```python
from build123d import *

# Parameters (mm, degrees)
SKETCH_1_W          = 13.6
SKETCH_1_H          = 5
EXTRUDE_1_DEPTH     = 1.2
SKETCH_2_W          = 1.2
SKETCH_2_H          = 5
EXTRUDE_2_DEPTH     = 5
SKETCH_3_R          = 1
CUT_EXTRUDE_1_DEPTH = 14
SKETCH_5_W          = 1.2
SKETCH_5_H          = 5
EXTRUDE_3_DEPTH     = 2


with BuildPart() as part:
    # 草图1 → 凸台-拉伸1 (new body)
    with BuildSketch(Plane.XY):
        with Locations((8.287992891, 2.5)):
            Rectangle(SKETCH_1_W, SKETCH_1_H)
    extrude(amount=EXTRUDE_1_DEPTH)

    # 草图2 → 凸台-拉伸2 (add)
    with BuildSketch(Plane(origin=(0, 0, 1.2), x_dir=(-1, 0, 0), z_dir=(0, 0, -1))):
        with Locations((-14.487992891, 2.5)):
            Rectangle(SKETCH_2_W, SKETCH_2_H)
        with Locations((-2.087992891, 2.5)):
            Rectangle(SKETCH_2_W, SKETCH_2_H)
    extrude(amount=-EXTRUDE_2_DEPTH)

    # 草图3 → 切除-拉伸1 (cut)
    with BuildSketch(Plane(origin=(15.087992891, 0, 0), x_dir=(0, 0, -1), z_dir=(1, 0, 0))):
        with Locations((-4, 2.5)):
            Circle(SKETCH_3_R)
    extrude(amount=-CUT_EXTRUDE_1_DEPTH, mode=Mode.SUBTRACT)

    # 草图5 → 凸台-拉伸3 (add)
    with BuildSketch(Plane(origin=(0, 0, 0), x_dir=(-1, 0, 0), z_dir=(0, 0, -1))):
        with Locations((-2.087992891, 2.5)):
            Rectangle(SKETCH_5_W, SKETCH_5_H)
    extrude(amount=EXTRUDE_3_DEPTH)


solid = part.part
```
Build history of the part. All positions in model axes, mm. A direction names the side the tool comes from. Give positions to 0.01 mm unless a question says otherwise; leave off trailing zeros. Loops run counter-clockwise (first coordinate to the right, second up) from the corner with the lowest first, then second, coordinate; pieces in that order, holes last. Notation, with made-up numbers: (-14.5, 15.25) - (19.5, 15.25) arc R21 ccw to (19.5, 34.25) - close; hole circle Ø10 at (68.5, -12). An arc over 180 degrees is marked (long way). Use a Markdown table: item, result.
(1) Band-saw the part on A-A (y = 2.5). Give the cut face in (x, z), and give its area (3 significant figures).
Taken from the geometry:
| item | result |
|---|---|
| outline | (1.49, -2) - (2.69, -2) - (2.69, 0) - (15.09, 0) - (15.09, 3) - (13.89, 3) - (13.89, 1.2) - (2.69, 1.2) - (2.69, 3) - (1.49, 3) - close; (1.49, 5) - (2.69, 5) - (2.69, 6.2) - (1.49, 6.2) - close; (13.89, 5) - (15.09, 5) - (15.09, 6.2) - (13.89, 6.2) - close |
| area | 25.9 mm2 |
(2) Wall check: line 1 along X through (y, z) = (2.65, 2.5); line 2 along Y through (x, z) = (14.7, 4); line 3 along Z through (x, y) = (12.25, 0.3). Give the ranges that are in metal, low to high.
Taken from the geometry:
| item | result |
|---|---|
| line 1 | 1.49 to 2.69, 13.89 to 15.09 |
| line 2 | 0 to 1.5, 3.5 to 5 |
| line 3 | 0 to 1.2 |
(3) Band-saw the part on B-B (z = 4). Give the cut face in (x, y).
Taken from the geometry:
| item | result |
|---|---|
| outline | (1.49, 0) - (2.69, 0) - (2.69, 1.5) - (1.49, 1.5) - close; (1.49, 3.5) - (2.69, 3.5) - (2.69, 5) - (1.49, 5) - close; (13.89, 0) - (15.09, 0) - (15.09, 1.5) - (13.89, 1.5) - close; (13.89, 3.5) - (15.09, 3.5) - (15.09, 5) - (13.89, 5) - close |
(4) Which spindle directions (+Z, -Z, +X, -X, +Y, -Y) get a long thin tool onto all of the face, cutting with end or side? Do faces 1 (the face through (8, 3, 1.2)), 2 (the face through (15.088, 2, 2)), 3 (the face through (2.688, 2, -1)). Say none if no direction does.
Taken from the geometry:
| item | result |
|---|---|
| face 1 | +Z, +Y, -Y |
| face 2 | +Z, -Z, +X, +Y, -Y |
| face 3 | -Z, +X, +Y, -Y |
(5) Drop flat-ended pins along their axis: pin 1 Ø2.5 at (x, y) = (8, 1.5) entering from +Z; pin 2 Ø2.5 at (x, y) = (9.5, 3.5) entering from -Z; pin 3 Ø1 at (y, z) = (2.5, -1.5) entering from +X; pin 4 Ø1.6 at (y, z) = (2.5, 4) entering from -X. Give the stop position or say it passes through.
Taken from the geometry:
| item | result |
|---|---|
| pin 1 | z = 1.2 |
| pin 2 | z = 0 |
| pin 3 | x = 2.69 |
| pin 4 | through |
(6) Pull direction Z, two halves, no side cores. Call faces 4 (the face through (13.888, 2.5, 2.6)), 5 (the face through (2.1, 2.5, 5)), 6 (the face through (9, 3, 0)): +Z half, -Z half, draft (parallel to the pull), parting line (faces both ways), or undercut.
Taken from the geometry:
| item | result |
|---|---|
| face 4 | draft |
| face 5 | undercut |
| face 6 | -Z half |
(7) Band-saw the part on C-C (z = 2.5). Give the cut face in (x, y), and give its area (3 significant figures).
Taken from the geometry:
| item | result |
|---|---|
| outline | (1.49, 0) - (2.69, 0) - (2.69, 5) - (1.49, 5) - close; (13.89, 0) - (15.09, 0) - (15.09, 5) - (13.89, 5) - close |
| area | 12.0 mm2 |
(8) Band-saw the part on D-D (y = 3.7). Give the cut face in (x, z), and give its area (3 significant figures).
Taken from the geometry:
| item | result |
|---|---|
| outline | (1.49, -2) - (2.69, -2) - (2.69, 0) - (15.09, 0) - (15.09, 6.2) - (13.89, 6.2) - (13.89, 1.2) - (2.69, 1.2) - (2.69, 6.2) - (1.49, 6.2) - close |
| area | 30.7 mm2 |
